Design review of the part shown in the three views and the two pictorial views. Dimensions are in mm from the part's minimum x, y and z. Give positions to 0.01 mm unless a question says otherwise; leave off trailing zeros. Order: outer loops, then holes, each group sorted by start corner. A loop starts at its lowest first (then second) coordinate and runs counter-clockwise, first axis right, second up. Notation, with made-up numbers: (-19.75, -16) - (24.25, -16) arc R10 cw to (24.25, 1) - close; hole circle Ø11 at (-32, -14.75). An arc over 180 degrees is marked (long way). Put each result on its own line as item: value.
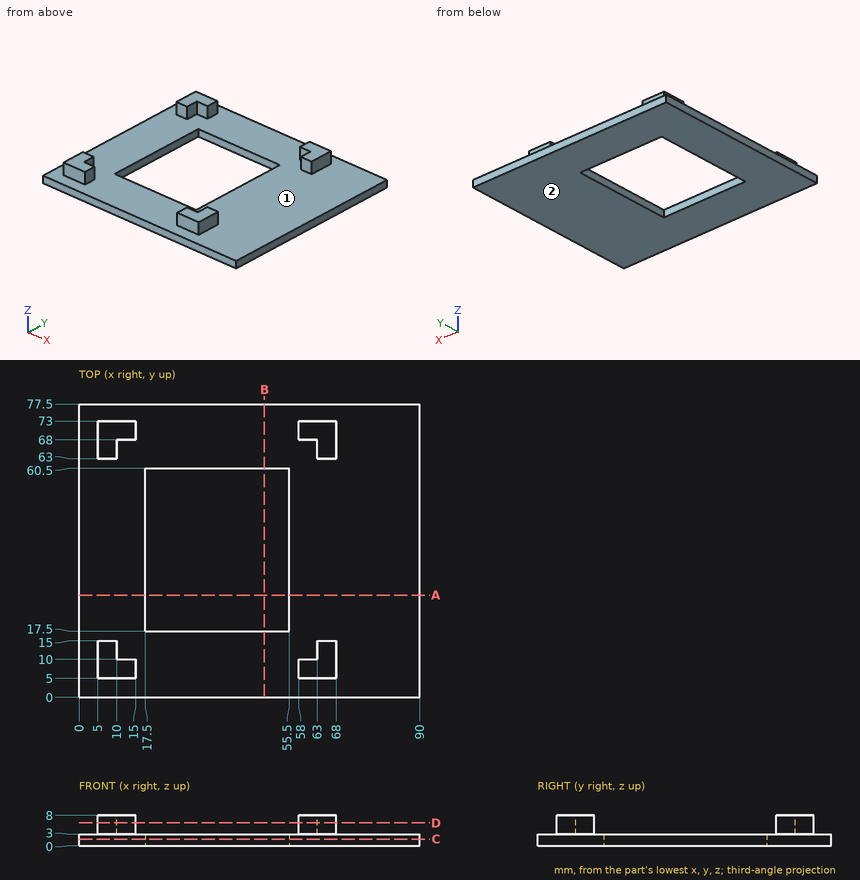
(1) Wall thickness on L1, parallel to X at y = 66.5, z = 5.75; L2, parallel to Y at x = 21.5, z = 2.25; L3, parallel to Y at x = 7, z = 5: over which ranges is each line inside the solid? List them lowest first.
The answers:
L1: 5 to 10, 63 to 68
L2: 0 to 17.5, 60.5 to 77.5
L3: 5 to 15, 63 to 73
(2) The part is to be moulded in two halves that separate along X. For the marked faces 1 and 2, say which applies: pulls with the +X half, pulls with the -X half, needs draft (parallel to the pull), parting line crosses it, or undercut.
The answers:
face 1: undercut
face 2: needs draft
(3) Take a section at C-C, the plane z = 1.75. Write out the cut boundary in (x, y).
The answers:
outline: (0, 0) - (90, 0) - (90, 77.5) - (0, 77.5) - close; hole (17.5, 17.5) - (55.5, 17.5) - (55.5, 60.5) - (17.5, 60.5) - close
(4) Clearance check with flat-ended pins moving along their axes: pin 1 Ø1.5 at (x, y) = (66.5, 48.5) entering from -Z; pin 2 Ø1.5 at (y, z) = (65.5, 4.5) entering from +X; pin 3 Ø2.5 at (y, z) = (69.5, 6.5) entering from -X; pin 4 Ø1.5 at (x, y) = (72, 62) entering from +Z. State where each tip first meets the part, or that it passes through.
The answers:
pin 1: z = 0
pin 2: x = 68
pin 3: x = 5
pin 4: z = 3
(5) Take a section at A-A, the plane y = 27. Write out the cut boundary in (x, z), then the cut area to 3 significant figures.
The answers:
outline: (0, 0) - (17.5, 0) - (17.5, 3) - (0, 3) - close; (55.5, 0) - (90, 0) - (90, 3) - (55.5, 3) - close
area: 156 mm^2
(6) Take a section at B-B, the plane x = 49. Write out the cut boundary in (y, z), then the cut area to 4 significant figures.
The answers:
outline: (0, 0) - (17.5, 0) - (17.5, 3) - (0, 3) - close; (60.5, 0) - (77.5, 0) - (77.5, 3) - (60.5, 3) - close
area: 103.5 mm^2
(7) Take a section at D-D, the plane z = 6. Write out the cut boundary in (x, y).
The answers:
outline: (5, 5) - (15, 5) - (15, 10) - (10, 10) - (10, 15) - (5, 15) - close; (5, 63) - (10, 63) - (10, 68) - (15, 68) - (15, 73) - (5, 73) - close; (58, 5) - (68, 5) - (68, 15) - (63, 15) - (63, 10) - (58, 10) - close; (58, 68) - (63, 68) - (63, 63) - (68, 63) - (68, 73) - (58, 73) - close
